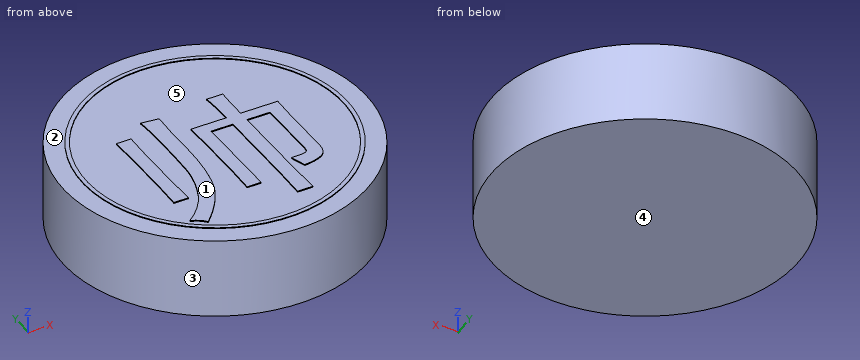
```python
from build123d import *

# Parameters (mm, degrees)
SKETCH_1_R               = 15
DIAMETER30_HEIGHT8_DEPTH = 8
CHARACTER_DEPTH          = 0.1
SKETCH_3_R               = 13.1
SKETCH_3_R_2             = 12.7
INK_RING_DEPTH           = 0.08


with BuildPart() as part:
    # 草图1 → Diameter30_Height8 (new body)
    with BuildSketch(Plane.XY):
        Circle(SKETCH_1_R)
    extrude(amount=-DIAMETER30_HEIGHT8_DEPTH)

    # 草图2 → Character_帅 (add)
    with BuildSketch(Plane.XY):
        with BuildLine():
            add(Edge.make_bspline(
                [(2.649122807, 2.657894737), (2.648277509, 2.838961546), (2.646647548, 3.188106947), (2.643949337, 3.693304246), (2.627710858, 4.161013978), (2.618261471, 4.592706352), (2.59561766, 4.986803608), (2.573364544, 5.343905172), (2.545932395, 5.6629896), (2.520624442, 5.862638482), (2.50877193, 5.956140351)],
                knots=[0, 0, 0, 0, 1.315583411, 2.536797873, 3.670260287, 4.715635349, 5.673736592, 6.537953599, 7.315277556, 8, 8, 8, 8], degree=3))
            Line((2.50877193, 5.956140351), (4.122807018, 5.956140351))
            add(Edge.make_bspline(
                [(4.122807018, 5.956140351), (4.117499898, 5.877309705), (4.105781963, 5.703254378), (4.089167905, 5.417436401), (4.081123846, 5.081109437), (4.069497803, 4.693902375), (4.062208699, 4.256354693), (4.058010495, 3.768573009), (4.051072159, 3.230576781), (4.052096052, 2.854561793), (4.052631579, 2.657894737)],
                knots=[0, 0, 0, 0, 0.574688494, 1.268892212, 2.082186167, 3.021459211, 4.086593269, 5.265055303, 6.569542337, 8, 8, 8, 8], degree=3))
            Line((4.052631579, 2.657894737), (7.771929825, 2.657894737))
            add(Edge.make_bspline(
                [(7.771929825, 2.657894737), (7.760796072, 2.449999982), (7.73890673, 2.041271737), (7.719157498, 1.435549924), (7.705407242, 0.848123825), (7.702957274, 0.461670931), (7.701754386, 0.271929825)],
                knots=[0, 0, 0, 0, 1.046485867, 2.057427233, 3.046233291, 4, 4, 4, 4], degree=3))
            Line((7.701754386, 0.271929825), (7.701754386, -4.850877193))
            add(Edge.make_bspline(
                [(7.701754386, -4.850877193), (7.700509851, -4.946341409), (7.69812364, -5.129379766), (7.659319509, -5.390999722), (7.605347303, -5.628411903), (7.522536164, -5.840237206), (7.420768732, -6.029019154), (7.289859981, -6.189160821), (7.140756422, -6.328733562), (6.901013102, -6.472408104), (6.563626246, -6.612761018), (6.121927666, -6.749793211), (5.6299881, -6.842128832), (5.284963987, -6.870952514), (5.105263158, -6.885964912)],
                knots=[0, 0, 0, 0, 0.91195479, 1.748536932, 2.524193789, 3.235017793, 3.917413987, 4.565660724, 5.204897301, 5.860042995, 7.225363373, 8.690313679, 10.276197647, 12, 12, 12, 12], degree=3))
            add(Edge.make_bspline(
                [(5.105263158, -6.885964912), (5.030622329, -6.645449861), (4.877118075, -6.150813287), (4.703323003, -5.662931781), (4.614035088, -5.412280702)],
                knots=[0, 0, 0, 0, 0.972491982, 2, 2, 2, 2], degree=3))
            add(Edge.make_bspline(
                [(4.614035088, -5.412280702), (4.703272413, -5.411616614), (4.873964221, -5.410346357), (5.116579774, -5.405384501), (5.334043291, -5.397378419), (5.526579613, -5.38822529), (5.693812444, -5.372515338), (5.836088174, -5.354724862), (5.952359909, -5.334162259), (6.04894766, -5.312443399), (6.128856661, -5.275644675), (6.193160306, -5.21721386), (6.247720931, -5.142694696), (6.295806352, -5.050517957), (6.327140956, -4.938045189), (6.350107, -4.808315534), (6.366009975, -4.660655055), (6.367588242, -4.555491891), (6.368421053, -4.5)],
                knots=[0, 0, 0, 0, 1.810479571, 3.463057961, 4.922871987, 6.225442376, 7.372781237, 8.329861336, 9.133212, 9.768407665, 10.334419243, 10.894946083, 11.510128595, 12.201898471, 12.991479159, 13.867141808, 14.874545699, 16, 16, 16, 16], degree=3))
            Line((6.368421053, -4.5), (6.368421053, 1.535087719))
            Line((6.368421053, 1.535087719), (4.052631579, 1.535087719))
            Line((4.052631579, 1.535087719), (4.052631579, -6.815789474))
            add(Edge.make_bspline(
                [(4.052631579, -6.815789474), (4.053765197, -7.103428128), (4.056001813, -7.670936452), (4.069634056, -8.508736417), (4.088763125, -9.320656714), (4.11158118, -9.852421744), (4.122807018, -10.114035088)],
                knots=[0, 0, 0, 0, 1.046194404, 2.064131589, 3.047607535, 4, 4, 4, 4], degree=3))
            Line((4.122807018, -10.114035088), (2.578947368, -10.114035088))
            add(Edge.make_bspline(
                [(2.578947368, -10.114035088), (2.590173206, -9.852421744), (2.612991261, -9.320656714), (2.63212033, -8.508736417), (2.645752573, -7.670936452), (2.647989189, -7.103428128), (2.649122807, -6.815789474)],
                knots=[0, 0, 0, 0, 0.952392465, 1.935868411, 2.953805596, 4, 4, 4, 4], degree=3))
            Line((2.649122807, -6.815789474), (2.649122807, 1.535087719))
            Line((2.649122807, 1.535087719), (0.473684211, 1.535087719))
            Line((0.473684211, 1.535087719), (0.473684211, -7.377192982))
            Line((0.473684211, -7.377192982), (-0.929824561, -7.377192982))
            add(Edge.make_bspline(
                [(-0.929824561, -7.377192982), (-0.918712527, -7.137237676), (-0.89705509, -6.669562974), (-0.877305751, -5.985025613), (-0.863382791, -5.336096743), (-0.860869477, -4.914994784), (-0.859649123, -4.710526316)],
                knots=[0, 0, 0, 0, 1.08047164, 2.105847367, 3.080283338, 4, 4, 4, 4], degree=3))
            Line((-0.859649123, -4.710526316), (-0.859649123, 0.271929825))
            add(Edge.make_bspline(
                [(-0.859649123, 0.271929825), (-0.860778179, 0.479865427), (-0.863003576, 0.889711309), (-0.876691761, 1.495334741), (-0.895801581, 2.082918827), (-0.918599793, 2.468200268), (-0.929824561, 2.657894737)],
                knots=[0, 0, 0, 0, 1.045182189, 2.060078265, 3.044873733, 4, 4, 4, 4], degree=3))
            Line((-0.929824561, 2.657894737), (2.649122807, 2.657894737))
        make_face()
        with BuildLine():
            add(Edge.make_bspline(
                [(-2.543859649, 5.394736842), (-2.55453691, 5.241410089), (-2.576968973, 4.919282974), (-2.606332671, 4.4133937), (-2.625722602, 3.862230343), (-2.641455489, 3.266150249), (-2.651530629, 2.625004365), (-2.656494342, 1.938824334), (-2.656719765, 1.207587715), (-2.649857053, 0.442624259), (-2.646120363, -0.33291913), (-2.667300728, -1.096525685), (-2.709346485, -1.836581392), (-2.767619156, -2.554468791), (-2.849443973, -3.249377344), (-2.946107025, -3.921647543), (-3.067303461, -4.570685232), (-3.204881304, -5.204412609), (-3.386965023, -5.831459902), (-3.6329141, -6.458227284), (-3.948908402, -7.087582997), (-4.324035754, -7.726937374), (-4.768016313, -8.370052347), (-5.274742334, -9.020901708), (-5.843502049, -9.679758443), (-6.259926358, -10.105844174), (-6.473684211, -10.324561404)],
                knots=[0, 0, 0, 0, 0.659190093, 1.384905098, 2.173195898, 3.024385089, 3.942285353, 4.923260466, 5.96737447, 7.078396075, 8.204255659, 9.293363896, 10.354008229, 11.383098418, 12.381857005, 13.354528352, 14.295395268, 15.213084928, 16.134880166, 17.092610712, 18.096292209, 19.152239996, 20.269451564, 21.445260402, 22.688607657, 24, 24, 24, 24], degree=3))
            add(Edge.make_bspline(
                [(-6.473684211, -10.324561404), (-6.559732909, -10.223409926), (-6.732267206, -10.020593389), (-7.051816717, -9.772809488), (-7.40742211, -9.558009314), (-7.671581713, -9.461672847), (-7.807017544, -9.412280702)],
                knots=[0, 0, 0, 0, 0.970214787, 1.94535571, 2.94657452, 4, 4, 4, 4], degree=3))
            add(Edge.make_bspline(
                [(-7.807017544, -9.412280702), (-7.657973182, -9.300088741), (-7.363260789, -9.078246324), (-6.955815499, -8.710596291), (-6.57424992, -8.328429932), (-6.223348035, -7.926246582), (-5.904578485, -7.503232626), (-5.618396742, -7.059527971), (-5.360624691, -6.597131501), (-5.135263603, -6.115997615), (-4.940375439, -5.623171603), (-4.765347571, -5.126552857), (-4.614790167, -4.626941063), (-4.485965447, -4.124417421), (-4.385577394, -3.617432725), (-4.307679883, -3.107532014), (-4.251338798, -2.595099135), (-4.218416323, -1.902922648), (-4.195596224, -1.026008016), (-4.174639454, 0.042281327), (-4.161380369, 1.13219518), (-4.159064793, 1.86603464), (-4.157894737, 2.236842105)],
                knots=[0, 0, 0, 0, 0.876110196, 1.73237371, 2.575729557, 3.4124282, 4.237942316, 5.062170833, 5.891260029, 6.723431221, 7.556418375, 8.38034529, 9.196777122, 10.007322445, 10.81680406, 11.623928264, 12.430374722, 13.237591303, 14.878759917, 16.552082939, 18.25777509, 20, 20, 20, 20], degree=3))
            add(Edge.make_bspline(
                [(-4.157894737, 2.236842105), (-4.158742697, 2.42310712), (-4.160379489, 2.782648704), (-4.163043616, 3.302572137), (-4.179306434, 3.783279411), (-4.188638552, 4.224503155), (-4.21144322, 4.62552561), (-4.233545861, 4.986968321), (-4.261113513, 5.309505904), (-4.286397635, 5.510893979), (-4.298245614, 5.605263158)],
                knots=[0, 0, 0, 0, 1.325220203, 2.558031484, 3.6987413, 4.747031617, 5.69752876, 6.556083798, 7.323389997, 8, 8, 8, 8], degree=3))
            add(Edge.make_bspline(
                [(-4.298245614, 5.605263158), (-4.138880204, 5.583255195), (-3.828993721, 5.54046065), (-3.377518369, 5.48397261), (-2.952393963, 5.432706182), (-2.677341911, 5.407142736), (-2.543859649, 5.394736842)],
                knots=[0, 0, 0, 0, 1.092444961, 2.124262261, 3.089707881, 4, 4, 4, 4], degree=3))
        make_face()
        with BuildLine():
            add(Edge.make_bspline(
                [(-6.192982456, 3.921052632), (-6.213127144, 3.470616313), (-6.25390666, 2.558784097), (-6.260049539, 1.646058489), (-6.263157895, 1.184210526)],
                knots=[0, 0, 0, 0, 0.987980705, 2, 2, 2, 2], degree=3))
            Line((-6.263157895, 1.184210526), (-6.263157895, -3.51754386))
            add(Edge.make_bspline(
                [(-6.263157895, -3.51754386), (-6.262026133, -3.760132755), (-6.259790748, -4.239279455), (-6.246045202, -4.949726115), (-6.226937452, -5.6429749), (-6.204202458, -6.099339702), (-6.192982456, -6.324561404)],
                knots=[0, 0, 0, 0, 1.036632017, 2.04749195, 3.036413013, 4, 4, 4, 4], degree=3))
            Line((-6.192982456, -6.324561404), (-7.666666667, -6.324561404))
            add(Edge.make_bspline(
                [(-7.666666667, -6.324561404), (-7.655523902, -6.083740603), (-7.633604379, -5.610009217), (-7.61410139, -4.912465947), (-7.600135574, -4.241012646), (-7.597689835, -3.802584211), (-7.596491228, -3.587719298)],
                knots=[0, 0, 0, 0, 1.05657797, 2.078450635, 3.058287504, 4, 4, 4, 4], degree=3))
            Line((-7.596491228, -3.587719298), (-7.596491228, 1.254385965))
            add(Edge.make_bspline(
                [(-7.596491228, 1.254385965), (-7.597623519, 1.485712467), (-7.599858589, 1.94233606), (-7.613556549, 2.618130935), (-7.632693155, 3.27586782), (-7.655445944, 3.707961922), (-7.666666667, 3.921052632)],
                knots=[0, 0, 0, 0, 1.040483654, 2.053847617, 3.040239174, 4, 4, 4, 4], degree=3))
            Line((-7.666666667, 3.921052632), (-6.192982456, 3.921052632))
        make_face()
    extrude(amount=CHARACTER_DEPTH)

    # 草图3 → Ink_ring (add)
    with BuildSketch(Plane.XY):
        with Locations(Location((0, 0, 0), (0, 0, 180))):
            Circle(SKETCH_3_R)
        with Locations(Location((0, 0, 0), (0, 0, 180))):
            Circle(SKETCH_3_R_2, mode=Mode.SUBTRACT)
    extrude(amount=INK_RING_DEPTH)


solid = part.part
```
Verification items for the finished model (mm, model axes). Face numbers are marked on the shaded views. A direction names the side the tool comes from. Coordinates: 2 decimals unless noted, no trailing zeros. Loops run counter-clockwise (first coordinate to the right, second up) from the corner with the lowest first, then second, coordinate; pieces in that order, holes last. Notation, with made-up numbers: (63, 9.5) - (107, 9.5) arc R26 cw to (107, 44.5) - close; hole circle Ø3 at (-22.75, 45.25). An arc over 180 degrees is marked (long way). Answer as a JSON object with one key per item and string values.
(1) Mould release check, pull along Y, two halves, no side actions. Record for the marked faces 3, 4 and 5: pulls with the +Y half, pulls with the -Y half, needs draft (parallel to the pull), parting line crosses it, or undercut.
Response:
{"face 3": "parting line crosses it", "face 4": "needs draft", "face 5": "undercut"}
(2) Scan lines: line 1 along Z through (x, y) = (-11.75, -8.25); line 2 along Z through (x, y) = (-1.25, -13); line 3 along Y through (x, z) = (-10.25, -7). Record each from-to range of solid material in increasing order.
Response:
{"line 1": "z = -8 to 0", "line 2": "z = -8 to 0.08", "line 3": "y = -10.95 to 10.95"}
(3) Go/stop test with flat-tipped pins: pin 1 Ø3 at (x, y) = (10, 4) entering from +Z; pin 2 Ø4 at (x, z) = (5, -1) entering from +Y; pin 3 Ø2 at (y, z) = (-10, -2.5) entering from -X. Record where each tip stops, or that it passes through.
Response:
{"pin 1": "stops at z = 0", "pin 2": "stops at y = 14.7", "pin 3": "stops at x = -12"}
(4) Cross-section at A-A, the plane x = 2. Record the boundary of the cut face in (y, z), then the cut area to 3 significant figures.
Response:
{"outline": "(-14.87, -8) - (14.87, -8) - (14.87, 0) - (12.95, 0) - (12.95, 0.08) - (12.54, 0.08) - (12.54, 0) - (2.66, 0) - (2.66, 0.1) - (1.54, 0.1) - (1.54, 0) - (-12.54, 0) - (-12.54, 0.08) - (-12.95, 0.08) - (-12.95, 0) - (-14.87, 0) - close", "area": "238 mm²"}
(5) Access from +Z, -Z, +X, -X, +Y, -Y to the whole of each face (thin tool, end or side, straight path). Record for the marked faces 1 and 2.
Response:
{"face 1": "+Z, +X, -X, +Y, -Y", "face 2": "+Z"}
(6) Cross-section at C-C, the plane x = 9.75. Record the boundary of the cut face in (y, z), then the cut area to 3 significant figures.
Response:
{"outline": "(-11.4, -8) - (11.4, -8) - (11.4, 0) - (8.75, 0) - (8.75, 0.08) - (8.14, 0.08) - (8.14, 0) - (-8.14, 0) - (-8.14, 0.08) - (-8.75, 0.08) - (-8.75, 0) - (-11.4, 0) - close", "area": "182 mm²"}
(7) Cross-section at B-B, the plane z = -2.5. Record the boundary of the cut face in (x, y), then the cut area to 3 significant figures.
Response:
{"outline": "circle Ø30 at (0, 0)", "area": "707 mm²"}
